Autodesk Inventor part; units mm, degrees
ref_plane "Piano di lavoro9" through (123.3139, -0.0528, 92.5382) normal (1, 0, 0) x (0, 0, -1)
ref_plane "Piano di lavoro11" through (123.3139, -0.0528, 92.5382) normal (1, 0, 0) x (0, 0, -1)
ref_plane "YZ Plane" through (0, 0, 0) normal (1, 0, 0) x (0, 1, 0)
ref_plane "Piano di lavoro9" through (123.3139, -0.0528, 92.5382) normal (1, 0, 0) x (0, 0, -1)
sketch "Schizzo5" plane through (123.3139, -0.0528, 92.5382) normal (1, 0, 0) x (0, 0, -1)
  line L0 (71.3231, 66.1847) -> (134.8231, 66.1847)
  line L1 (134.8231, 66.1847) -> (134.8231, 34.6847)
  line L2 (134.8231, 34.6847) -> (71.3231, 34.6847)
  line L3 (71.3231, 34.6847) -> (71.3231, 66.1847)
  line L4 (71.3231, 34.6847) -> (81.3231, 34.6847)
  line L5 (81.3231, 34.6847) -> (81.3231, 29.6847)
  line L6 (81.3231, 29.6847) -> (71.3231, 29.6847)
  line L7 (134.8231, 34.6847) -> (124.8231, 34.6847)
  line L8 (124.8231, 34.6847) -> (124.8231, 29.6847)
  line L9 (124.8231, 29.6847) -> (134.8231, 29.6847)
  line L10 (71.3231, 66.1847) -> (81.3231, 66.1847)
  line L11 (81.3231, 66.1847) -> (81.3231, 69.1847)
  line L12 (81.3231, 69.1847) -> (71.3231, 69.1847)
  line L13 (134.8231, 66.1847) -> (124.8231, 66.1847)
  line L14 (124.8231, 66.1847) -> (124.8231, 69.1847)
  line L15 (124.8231, 69.1847) -> (134.8231, 69.1847)
  line L16 (71.3231, 69.1847) -> (68.3231, 69.1847)
  line L17 (68.3231, 69.1847) -> (68.3231, 29.6847)
  line L18 (68.3231, 29.6847) -> (71.3231, 29.6847)
  line L19 (71.3231, 34.6847) -> (71.3231, 66.1847)
  line L20 (134.8231, 69.1847) -> (137.8231, 69.1847)
  line L21 (137.8231, 69.1847) -> (137.8231, 29.6847)
  line L22 (137.8231, 29.6847) -> (134.8231, 29.6847)
  point P0 (92.5382, 0.0528)
  dimension "d18" = 63.5
  dimension "d19" = 31.5
  dimension "d20" = 10
  dimension "d21" = 5
  dimension "d22" = 10
  dimension "d23" = 5
  dimension "d24" = 10
  dimension "d25" = 3
  dimension "d26" = 10
  dimension "d27" = 3
  dimension "d28" = 3
  dimension "d29" = 3
extrude "Estrusione3" add sketch "Schizzo5" against normal blind 100 contours L3 L2 L5 L6 L18 L17 L16 L12 L11 L0 | L14 L15 L20 L21 L22 L9 L8 L2 L1 L0
ref_plane "Piano di lavoro11" through (123.3139, -0.0528, 92.5382) normal (1, 0, 0) x (0, 0, -1)
sketch "Schizzo6" plane through (123.3139, -0.0528, 92.5382) normal (1, 0, 0) x (0, 0, -1)
  line L0 (71.3231, 66.1847) -> (81.3231, 66.1847)
  line L1 (81.3231, 34.6847) -> (71.3231, 34.6847)
  line L2 (81.3231, 29.6847) -> (81.3231, 34.6847)
  line L3 (134.8231, 66.1847) -> (134.8231, 34.6847)
  line L4 (71.3231, 34.6847) -> (71.3231, 66.1847)
  line L5 (68.3231, 99.6847) -> (137.155, 99.6847)
  line L6 (124.8231, 69.1847) -> (137.8231, 69.1847)
  line L7 (137.8231, 69.1847) -> (134.8231, 69.1847)
  line L8 (134.8231, 69.1847) -> (134.8231, 79.6847)
  line L9 (137.8231, 79.6847) -> (137.8231, 69.1847)
  line L10 (71.3231, 69.1847) -> (71.3231, 79.6847)
  line L11 (68.3231, 79.6847) -> (68.3231, 69.1847)
  line L12 (115.0731, 79.6847) -> (134.8231, 79.6847)
  line L13 (137.8231, 79.6847) -> (137.8231, 82.6847)
  line L14 (137.8231, 82.6847) -> (118.0731, 82.6847)
  line L15 (91.0731, 79.6847) -> (71.3231, 79.6847)
  line L16 (68.3231, 79.6847) -> (68.3231, 82.6847)
  line L17 (68.3231, 82.6847) -> (88.0731, 82.6847)
  line L18 (91.0731, 82.6847) -> (93.0731, 82.6847)
  line L19 (93.0731, 82.6847) -> (93.0731, 79.6847)
  line L20 (93.0731, 79.6847) -> (91.0731, 79.6847)
  line L21 (115.0731, 82.6847) -> (113.0731, 82.6847)
  line L22 (113.0731, 82.6847) -> (113.0731, 79.6847)
  line L23 (113.0731, 79.6847) -> (115.0731, 79.6847)
  line L24 (91.0731, 82.6847) -> (91.0731, 84.6847)
  line L25 (88.0731, 82.6847) -> (88.0731, 85.6847)
  line L26 (93.0731, 85.6847) -> (93.0731, 84.6847)
  line L27 (93.0731, 84.6847) -> (91.0731, 84.6847)
  line L28 (113.0731, 84.6847) -> (115.0731, 84.6847)
  line L29 (93.0731, 85.6847) -> (93.0731, 86.6847)
  line L30 (88.0731, 85.6847) -> (88.0731, 86.6847)
  line L31 (88.0731, 86.6847) -> (93.0731, 86.6847)
  line L32 (113.0731, 84.6847) -> (113.0731, 86.6847)
  line L33 (113.0731, 86.6847) -> (118.0731, 86.6847)
  line L34 (118.0731, 86.6847) -> (118.0731, 82.6847)
  line L35 (115.0731, 84.6847) -> (115.0731, 82.6847)
  line L36 (68.3231, 69.1847) -> (81.3231, 69.1847)
  line L37 (71.3231, 69.1847) -> (68.3231, 69.1847)
  point P0 (92.5382, 0.0528)
  point P1 (68.3231, 29.6847)
  dimension "d32" = 70
  dimension "d33" = 31.5
  dimension "d35" = 63.5
  dimension "d37" = 3
  dimension "d38" = 10.5
  dimension "d39" = 3
  dimension "d40" = 10.5
  dimension "d43" = 3
  dimension "d44" = 3
  dimension "d45" = 2
  dimension "d46" = 2
  dimension "d47" = 2
  dimension "d50" = 2
  dimension "d54" = 2
  dimension "d55" = 4
  dimension "d56" = 5
  dimension "d57" = 2
  dimension "d58" = 2
  dimension "d59" = 5
extrude "Estrusione4" add sketch "Schizzo6" against normal blind 50
sketch "Schizzo7" plane through (123.3139, 29.6319, -32.2849) normal (0, 0, 1) x (1, 0, 0)
  line L0 (0, 5) -> (0, 0)
  line L1 (0, 5) -> (-100, 5)
  line L2 (-100, 0) -> (-100, 5)
  line L3 (0, 0) -> (-100, 0)
  point P0 (-123.3139, -29.6319)
extrude "Estrusione5" add sketch "Schizzo7" along normal blind 47.25
sketch "Schizzo8" plane through (123.3139, -0.0528, 92.5382) normal (1, 0, 0) x (0, 0, -1)
  line L0 (71.3231, 66.1847) -> (71.3231, 34.6847)
  line L1 (71.3231, 34.6847) -> (65.0934, 34.6847)
  line L2 (134.8231, 34.6847) -> (141.848, 34.6847)
  line L3 (137.8231, 29.6847) -> (137.8231, 82.6847)
  line L4 (68.3231, 29.6847) -> (68.3231, 69.1847)
  line L5 (137.8231, 34.6847) -> (68.3231, 34.6847)
  line L6 (68.3231, 34.6847) -> (68.3231, 29.6797)
  line L7 (137.8231, 29.6797) -> (137.8231, 34.6847)
  line L8 (68.3231, 29.6847) -> (137.86, 29.6847)
  line L9 (93.0823, 34.6854) -> (113.0823, 34.6854)
  line L10 (113.0823, 34.6854) -> (113.0823, 29.6854)
  line L11 (113.0823, 29.6854) -> (93.0823, 29.6854)
  line L12 (93.0823, 29.6854) -> (93.0823, 34.6854)
  line L13 (113.0823, 34.6854) -> (93.0823, 34.6854)
  line L14 (93.0823, 34.6854) -> (93.0823, 29.6854)
  line L15 (93.0823, 29.6854) -> (113.0823, 29.6854)
  line L16 (113.0823, 29.6854) -> (113.0823, 34.6854)
  point P0 (92.5382, 0.0528)
  point P1 (103.0823, 32.1854)
  point P2 (103.0823, 32.1854)
  point P3 (113.0823, 34.6847)
  point P4 (93.0823, 34.6847)
  dimension "d82" = 20
  dimension "d83" = 5
extrude "Estrusione6" add sketch "Schizzo8" along normal blind 25 contours L5 L10 L8 L12
sketch "Schizzo9" plane through (23.3139, -0.0528, 92.5382) normal (-1, 0, 0) x (0, 0, 1)
  line L0 (-71.3231, 66.1847) -> (-71.3231, 34.6847)
  line L1 (-71.3231, 34.6847) -> (-67.9708, 34.6847)
  line L2 (-68.3231, 82.6847) -> (-68.3231, 29.6847)
  line L3 (-68.3231, 29.6847) -> (-137.8231, 29.6847)
  line L4 (-68.3231, 34.6847) -> (-137.8231, 34.6847)
  line L5 (-137.8231, 34.6847) -> (-137.8231, 29.6847)
  line L6 (-137.8231, 29.6847) -> (-68.3231, 29.6847)
  line L7 (-68.3231, 29.6847) -> (-68.3231, 34.6847)
  line L8 (-113.0731, 34.6847) -> (-93.0731, 34.6847)
  line L9 (-93.0731, 34.6847) -> (-93.0731, 29.6847)
  line L10 (-93.0731, 29.6847) -> (-113.0731, 29.6847)
  line L11 (-113.0731, 29.6847) -> (-113.0731, 34.6847)
  point P0 (-92.5382, 0.0528)
  point P1 (-103.0731, 32.1847)
  point P2 (-103.0731, 32.1847)
  dimension "d86" = 20
  dimension "d87" = 5
extrude "Estrusione7" add sketch "Schizzo9" along normal blind 25 contours L9 L3 L11 L4
sketch "Schizzo10" plane through (23.3139, 34.6319, 21.2151) normal (0, 1, 0) x (1, 0, 0)
  line L0 (-25, 21.75) -> (-25, 41.75)
  line L1 (-25, 31.75) -> (-20, 31.75)
  circle A0 centre (-20, 31.75) radius 0.5
  line L2 (125, 41.7592) -> (125, 21.7592)
  line L3 (125, 31.7592) -> (120, 31.7592)
  circle A1 centre (120, 31.7592) radius 0.5
  point P0 (-23.3139, 21.2151)
  dimension "d90" = 5
  dimension "d91" = 1
  dimension "d92" = 5
  dimension "d93" = 1
sketch "Schizzo11" plane through (148.3139, -0.0528, 92.5382) normal (1, 0, 0) x (0, 0, -1)
  line L0 (113.0823, 34.6847) -> (93.0823, 34.6847)
  line L1 (113.0823, 29.6854) -> (113.0823, 34.6847)
  line L2 (93.0823, 34.6847) -> (113.0823, 34.6847)
  line L3 (113.0823, 34.6847) -> (113.0823, 29.6854)
  line L4 (113.0823, 29.6854) -> (93.0823, 29.6854)
  line L5 (93.0823, 29.6854) -> (93.0823, 34.6847)
  point P0 (92.5382, 0.0528)
extrude "Estrusione8" add sketch "Schizzo11" along normal blind 5
sketch "Schizzo12" plane through (-1.6861, -0.0528, 92.5382) normal (-1, 0, 0) x (0, 0, 1)
  line L0 (-113.0731, 34.6847) -> (-134.8231, 34.6847)
  line L1 (-113.0823, 29.6854) -> (-93.0823, 29.6854)
  line L2 (-113.0731, 34.6847) -> (-93.0823, 34.6847)
  line L3 (-93.0823, 34.6847) -> (-93.0823, 29.6854)
  line L4 (-93.0823, 29.6854) -> (-113.0731, 29.6854)
  line L5 (-113.0731, 29.6854) -> (-113.0731, 34.6847)
  point P0 (-92.5382, 0.0528)
extrude "Estrusione9" add sketch "Schizzo12" along normal blind 5
hole "Foro3" at (-1.6861, 34.6319, -10.5349) direction (0, -1, 0) diameter 3 end through all countersink diameter 4 countersink angle 90
sketch "Schizzo13" plane through (23.3139, 34.6319, 21.2151) normal (0, 1, 0) x (1, 0, 0)
  line L0 (130, 41.7592) -> (130, 21.7592)
  line L1 (130, 31.7592) -> (125, 31.7592)
  point P0 (-23.3139, 21.2151)
  dimension "d133" = 5
hole "Foro4" at (148.3139, 34.6319, -10.5442) direction (0, -1, 0) diameter 3 end through all countersink diameter 4 countersink angle 90
properties part number "pignat_2_Stampa 3D"
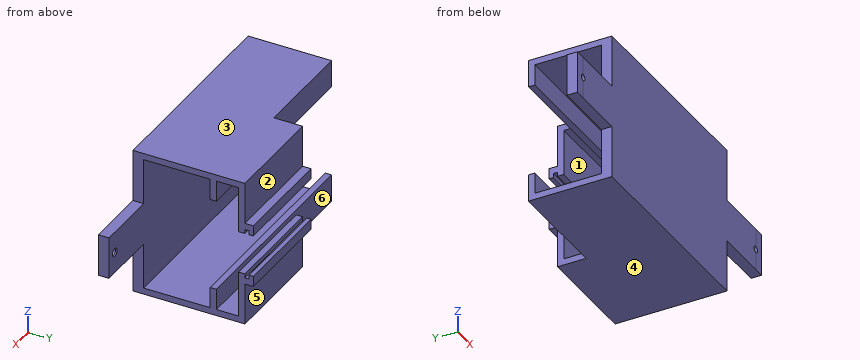
Can you work these out from the model? Positions are in its coordinate system, mm. Face numbers are marked on the shaded views. A direction names the side the tool comes from. Coordinates: 2 decimals unless noted, no trailing zeros. Order: outer loops, then holes, each group sorted by start corner. A loop starts at its lowest first (then second) coordinate and runs counter-clockwise, first axis right, second up. Notation, with made-up numbers: (85.5, 37.25) -> (132.5, 37.25) arc R6 ccw to (132.5, 44.25) -> close; hole circle Ø5 at (-20, 41). An arc over 180 degrees is marked (long way). Use one line per item in the form item = value.
Q1. We'd pull the mould along Z, two halves only. Please class the marked faces 3, 4, 5 and 6: released by +Z, released by -Z, zero draft, split by the parting line, or undercut.
From the geometry:
face_3 = released by +Z
face_4 = released by -Z
face_5 = zero draft
face_6 = undercut
Q2. Imagine slicing it at D-D, the plane x = 59. List the corners of the cut face in (y, z) for me.
From the geometry:
outline = (29.63, -45.28) -> (69.13, -45.28) -> (69.13, -32.28) -> (66.13, -32.28) -> (66.13, -42.28) -> (34.63, -42.28) -> (34.63, 21.22) -> (66.13, 21.22) -> (66.13, 11.22) -> (69.13, 11.22) -> (69.13, 24.22) -> (29.63, 24.22) -> close
Q3. I need wall thicknesses on L1, parallel to Y at x = 89, z = 0; L2, parallel to Y at x = 116, z = 20; L3, parallel to Y at x = 89, z = -30. Which ranges of each line are inside material? Lowest first, please.
From the geometry:
L1 = 29.63 to 34.63, 79.63 to 82.63, 84.63 to 86.63
L2 = 29.63 to 34.63, 66.13 to 69.13, 79.63 to 82.63
L3 = 29.63 to 34.63, 79.63 to 82.63
Q4. Will these pins go through, and if not, where does the flat tip stop? P1, Ø8, axis at x = 119, z = 8.5, coming from the +Y side; P2, Ø5.5, axis at x = 132.5, y = 31, coming from the +Z side; P3, Ø10, axis at y = 59.5, z = -33.5, coming from the +X side; P4, Ø4, axis at x = 13.5, z = -13, coming from the +Y side.
From the geometry:
P1 = 82.63
P2 = -0.54
P3 = through
P4 = 34.63
Q5. Imagine slicing it at B-B, the plane y = 48. List the corners of the cut face in (x, z) for me.
From the geometry:
outline = (23.31, -45.28) -> (123.31, -45.28) -> (123.31, -42.28) -> (23.31, -42.28) -> close; (23.31, 21.22) -> (123.31, 21.22) -> (123.31, 24.22) -> (23.31, 24.22) -> close
Q6. Which directions (+Z, -Z, +X, -X, +Y, -Y) give clear straight access to the entire face, cutting with the end or side of a thin tool? Please do the marked faces 1 and 2.
From the geometry:
face_1 = +X, -X
face_2 = +Z, +X, -X, +Y
Q7. Imagine slicing it at A-A, the plane z = -30. List the corners of the cut face in (x, y) for me.
From the geometry:
outline = (23.31, 29.63) -> (123.31, 29.63) -> (123.31, 34.63) -> (23.31, 34.63) -> close; (73.31, 79.63) -> (123.31, 79.63) -> (123.31, 82.63) -> (73.31, 82.63) -> close
